```python
from build123d import *
from build123d.topology import SkipClean

# Parameters (mm, degrees)
SKETCH1_W           = 36.97504
SKETCH1_H           = 88.55
SKETCH1_R           = 3.175
BOSS_EXTRUDE1_DEPTH = 3.5
BOSS_EXTRUDE3_START = 10.5
BOSS_EXTRUDE3_DEPTH = 10.5
CUT_EXTRUDE1_START  = 10.5
CUT_EXTRUDE1_DEPTH  = 10.5
SKETCH2_R           = 2.5
CUT_EXTRUDE2_DEPTH  = 3.5
FILLET1_R           = 2


with BuildPart() as part:
    # Sketch1 → Boss-Extrude1 (new body)
    with BuildSketch(Plane.XY):
        with Locations((18.48752, 44.275)):
            Rectangle(SKETCH1_W, SKETCH1_H)
        with Locations((31.575, 82.375)):
            Circle(SKETCH1_R, mode=Mode.SUBTRACT)
        with Locations((31.575, 56.975)):
            Circle(SKETCH1_R, mode=Mode.SUBTRACT)
        with Locations((31.575, 31.575)):
            Circle(SKETCH1_R, mode=Mode.SUBTRACT)
        with Locations((31.575, 6.175)):
            Circle(SKETCH1_R, mode=Mode.SUBTRACT)
        with Locations((6.175, 6.175)):
            Circle(SKETCH1_R, mode=Mode.SUBTRACT)
        with Locations((6.175, 31.575)):
            Circle(SKETCH1_R, mode=Mode.SUBTRACT)
        with Locations((6.175, 56.975)):
            Circle(SKETCH1_R, mode=Mode.SUBTRACT)
        with Locations((6.175, 82.375)):
            Circle(SKETCH1_R, mode=Mode.SUBTRACT)
    extrude(amount=-BOSS_EXTRUDE1_DEPTH)

    # Sketch1<4> → Boss-Extrude3 (add)
    with SkipClean():  # the faces are left unmerged after this step: merging them gives an invalid solid
        with BuildSketch(Plane.XY.offset(BOSS_EXTRUDE3_START)):
            with BuildLine():
                Line((33.47504, 0), (36.97504, 0))
                Line((36.97504, 0), (36.97504, 88.55))
                Line((36.97504, 88.55), (33.47504, 88.55))
                Line((33.47504, 88.55), (33.47504, 84.918712444))
                ThreePointArc((33.47504, 84.918712444), (34.75, 82.375), (33.47504, 79.831287556))
                Line((33.47504, 79.831287556), (33.47504, 59.518712444))
                ThreePointArc((33.47504, 59.518712444), (34.75, 56.975), (33.47504, 54.431287556))
                Line((33.47504, 54.431287556), (33.47504, 34.118712444))
                ThreePointArc((33.47504, 34.118712444), (34.75, 31.575), (33.47504, 29.031287556))
                Line((33.47504, 29.031287556), (33.47504, 8.718712444))
                ThreePointArc((33.47504, 8.718712444), (34.75, 6.175), (33.47504, 3.631287556))
                Line((33.47504, 3.631287556), (33.47504, 0))
            make_face()
        extrude(amount=-BOSS_EXTRUDE3_DEPTH)

    # Sketch1<5> → Cut-Extrude1 (cut)
    with BuildSketch(Plane.XY.offset(CUT_EXTRUDE1_START)):
        with BuildLine():
            ThreePointArc((36.25, 82.375), (35.495351515, 84.921854727), (33.47504, 86.646471994))
            Line((33.47504, 86.646471994), (33.47504, 84.918712444))
            ThreePointArc((33.47504, 84.918712444), (34.413419631, 83.797673188), (34.75, 82.375))
            ThreePointArc((34.75, 82.375), (34.413419631, 80.952326812), (33.47504, 79.831287556))
            Line((33.47504, 79.831287556), (33.47504, 78.103528006))
            ThreePointArc((33.47504, 78.103528006), (35.495351515, 79.828145273), (36.25, 82.375))
        make_face()
        with BuildLine():
            Line((33.47504, 84.918712444), (33.47504, 86.646471994))
            ThreePointArc((33.47504, 86.646471994), (26.9, 82.375), (33.47504, 78.103528006))
            Line((33.47504, 78.103528006), (33.47504, 79.831287556))
            ThreePointArc((33.47504, 79.831287556), (28.4, 82.375), (33.47504, 84.918712444))
        make_face()
        with BuildLine():
            ThreePointArc((36.25, 56.975), (35.495351515, 59.521854727), (33.47504, 61.246471994))
            Line((33.47504, 61.246471994), (33.47504, 59.518712444))
            ThreePointArc((33.47504, 59.518712444), (34.413419631, 58.397673188), (34.75, 56.975))
            ThreePointArc((34.75, 56.975), (34.413419631, 55.552326812), (33.47504, 54.431287556))
            Line((33.47504, 54.431287556), (33.47504, 52.703528006))
            ThreePointArc((33.47504, 52.703528006), (35.495351515, 54.428145273), (36.25, 56.975))
        make_face()
        with BuildLine():
            Line((33.47504, 59.518712444), (33.47504, 61.246471994))
            ThreePointArc((33.47504, 61.246471994), (26.9, 56.975), (33.47504, 52.703528006))
            Line((33.47504, 52.703528006), (33.47504, 54.431287556))
            ThreePointArc((33.47504, 54.431287556), (28.4, 56.975), (33.47504, 59.518712444))
        make_face()
        with BuildLine():
            ThreePointArc((33.47504, 35.846471994), (26.9, 31.575), (33.47504, 27.303528006))
            Line((33.47504, 27.303528006), (33.47504, 29.031287556))
            ThreePointArc((33.47504, 29.031287556), (28.4, 31.575), (33.47504, 34.118712444))
            Line((33.47504, 34.118712444), (33.47504, 35.846471994))
        make_face()
        with BuildLine():
            Line((33.47504, 29.031287556), (33.47504, 27.303528006))
            ThreePointArc((33.47504, 27.303528006), (35.495351515, 29.028145273), (36.25, 31.575))
            ThreePointArc((36.25, 31.575), (35.495351515, 34.121854727), (33.47504, 35.846471994))
            Line((33.47504, 35.846471994), (33.47504, 34.118712444))
            ThreePointArc((33.47504, 34.118712444), (34.413419631, 32.997673188), (34.75, 31.575))
            ThreePointArc((34.75, 31.575), (34.413419631, 30.152326812), (33.47504, 29.031287556))
        make_face()
        with BuildLine():
            ThreePointArc((33.47504, 10.446471994), (26.9, 6.175), (33.47504, 1.903528006))
            Line((33.47504, 1.903528006), (33.47504, 3.631287556))
            ThreePointArc((33.47504, 3.631287556), (28.4, 6.175), (33.47504, 8.718712444))
            Line((33.47504, 8.718712444), (33.47504, 10.446471994))
        make_face()
        with BuildLine():
            Line((33.47504, 3.631287556), (33.47504, 1.903528006))
            ThreePointArc((33.47504, 1.903528006), (35.495351515, 3.628145273), (36.25, 6.175))
            ThreePointArc((36.25, 6.175), (35.495351515, 8.721854727), (33.47504, 10.446471994))
            Line((33.47504, 10.446471994), (33.47504, 8.718712444))
            ThreePointArc((33.47504, 8.718712444), (34.413419631, 7.597673188), (34.75, 6.175))
            ThreePointArc((34.75, 6.175), (34.413419631, 4.752326812), (33.47504, 3.631287556))
        make_face()
    extrude(amount=-CUT_EXTRUDE1_DEPTH, mode=Mode.SUBTRACT)

    # Sketch2 → Cut-Extrude2 (cut)
    with BuildSketch(Plane(origin=(36.97504, 0, 0), x_dir=(0, 0, -1), z_dir=(1, 0, 0))):
        with Locations((-6.5, 17.849330816)):
            Circle(SKETCH2_R)
        with Locations((-6.5, 43.249330816)):
            Circle(SKETCH2_R)
        with Locations((-6.5, 68.649330816)):
            Circle(SKETCH2_R)
    extrude(amount=-CUT_EXTRUDE2_DEPTH, mode=Mode.SUBTRACT)

    # Fillet1
    fillet1_edges = [part.edges().sort_by_distance(p)[0] for p in [
        (33.47504, 44.275, 0),
        (33.47504, 18.875, 0),
        (33.47504, 0.951764003, 0),
        (33.47504, 87.598235997, 0),
        (33.47504, 69.675, 0),
    ]]
    fillet(fillet1_edges, radius=FILLET1_R)


solid = part.part
```
Geometry check sheet. Reference: the model listing, model coordinates, mm. A direction names the side the tool comes from. Round coordinates to 2 decimals unless told otherwise and drop trailing zeros. Write each loop counter-clockwise with the first axis right and the second up, starting at its lowest first coordinate (ties: lowest second). Pieces come first, ordered by that corner, then holes. Notation, with made-up numbers: (-2.75, 55) - (10.25, 55) arc R16 cw to (10.25, 77) - close; hole circle Ø7 at (-26.75, 40). An arc over 180 degrees is marked (long way). Write each question's results on one line, items separated by ' | '.
(1) Sectioned sample at D-D, the plane y = 22. Enter the section's corners in (x, z).
Computed:
outline: (0, -3.5) - (36.98, -3.5) - (36.98, 10.5) - (33.48, 10.5) - (33.48, 2) arc R2 cw to (31.48, 0) - (0, 0) - close
(2) Set-up check for faces 5 (the face through (5.487, 53.876, -1.726)), 6 (the face through (33.475, 72, 6)): record each of +Z, -Z, +X, -X, +Y, -Y from which the full face is reachable in a straight line by a thin tool's end or side.
Computed:
face 5: +Z, -Z | face 6: +Z, -X, +Y, -Y
(3) Sectioned sample at B-B, the plane y = 56. Enter the section's corners in (x, z), plus the area to 3 significant figures.
Computed:
outline: (0, -3.5) - (3.15, -3.5) - (3.15, 0) - (0, 0) - close; (9.2, -3.5) - (28.55, -3.5) - (28.55, 0) - (9.2, 0) - close; (34.6, -3.5) - (36.98, -3.5) - (36.98, 10.5) - (36.15, 10.5) - (36.15, 0) - (34.6, 0) - close | area: 95.8 mm^2
(4) Sectioned sample at C-C, the plane x = 5.5. Enter the section's corners in (y, z).
Computed:
outline: (0, -3.5) - (3.07, -3.5) - (3.07, 0) - (0, 0) - close; (9.28, -3.5) - (28.47, -3.5) - (28.47, 0) - (9.28, 0) - close; (34.68, -3.5) - (53.87, -3.5) - (53.87, 0) - (34.68, 0) - close; (60.08, -3.5) - (79.27, -3.5) - (79.27, 0) - (60.08, 0) - close; (85.48, -3.5) - (88.55, -3.5) - (88.55, 0) - (85.48, 0) - close
(5) Draft check along Y on faces 1 (the face through (35.25, 15.63, 5.35)), 2 (the face through (21, 88.55, -1)), 3 (the face through (30.887, 3.076, -1.726)), 4 (the face through (0, 44, -2)). Enter one of: pulls with the +Y half, pulls with the -Y half, needs draft (parallel to the pull), parting line crosses it, or undercut.
Computed:
face 1: undercut | face 2: pulls with the +Y half | face 3: undercut | face 4: needs draft
(6) Depth check by flat-ended pin: pin 1 Ø5.5 at (x, y) = (6.175, 31.575) entering from +Z; pin 2 Ø8.5 at (x, y) = (31.575, 6.175) entering from -Z; pin 3 Ø7 at (y, z) = (45.5, 5.5) entering from -X; pin 4 Ø2 at (y, z) = (54.5, 4) entering from -X. Enter the tip coordinate at first touch or a pass-through.
Computed:
pin 1: passes through | pin 2: stops at z = -3.5 | pin 3: stops at x = 33.48 | pin 4: stops at x = 34.7
(7) Thickness scan on probe 1 along Y at (x, z) = (33.5, -1); probe 2 along X at (y, z) = (30, -0.5); probe 3 along Z at (x, y) = (25.5, 14). Record the ranges inside material, lowest first. Write a range as from..to.
Computed:
probe 1: y = 0..3.65, 8.7..29.05, 34.1..54.45, 59.5..79.85, 84.9..88.55 | probe 2: x = 0..3.42, 8.93..28.82, 34.33..36.98 | probe 3: z = -3.5..0
(8) Sectioned sample at A-A, the plane z = 6.5. Enter the section's corners in (x, y) (3 decimals), plus the area to 3 significant figures.
Computed:
outline: (33.475, 0) - (36.975, 0) - (36.975, 15.349) - (33.475, 15.349) - (33.475, 10.446) arc R4.675 cw to (33.475, 1.904) - close; (33.475, 20.349) - (36.975, 20.349) - (36.975, 40.749) - (33.475, 40.749) - (33.475, 35.846) arc R4.675 cw to (33.475, 27.304) - close; (33.475, 45.749) - (36.975, 45.749) - (36.975, 66.149) - (33.475, 66.149) - (33.475, 61.246) arc R4.675 cw to (33.475, 52.704) - close; (33.475, 71.149) - (36.975, 71.149) - (36.975, 88.55) - (33.475, 88.55) - (33.475, 86.646) arc R4.675 cw to (33.475, 78.104) - close | area: 189 mm^2
